Job drawing, mm, ordinate dimensions from the low corner. One solid piece. Give positions to 0.01 mm unless a question says otherwise; leave off trailing zeros. Order: outer loops, then holes, each group sorted by start corner. A loop starts at its lowest first (then second) coordinate and runs counter-clockwise, first axis right, second up. Notation, with made-up numbers: (-31.5, 50.25) - (16.5, 50.25) arc R7 cw to (16.5, 57.25) - close; hole circle Ø1 at (-38.5, 34). An arc over 180 degrees is marked (long way). Use one line per item in the form item = value. Start each with the question number.
1. Pull direction Z, two halves, no side cores. Call the marked faces 1, 2 and 3: +Z half, -Z half, draft (parallel to the pull), parting line (faces both ways), or undercut.
2. Pin check, flat tips, straight feed: P1, Ø2.5, axis at x = 3.5, z = 61, coming from the -Y side; P2, Ø3, axis at x = 163, y = 16, coming from the +Z side. Stop position of each tip, or through.
3. Band-saw the part on A-A, the plane z = 101. List the corners of the cut face in (x, y).
4. Band-saw the part on B-B, the plane x = 135.5. List the corners of the cut face in (y, z), plus the area to 3 significant figures.
5. Band-saw the part on D-D, the plane y = 12. List the corners of the cut face in (x, z) (1 decimal), plus the area to 3 significant figures.
6. Drill centre lines: line 1 (X direction, y = 41, z = 54.5); line 2 (Z direction, x = 31.5, y = 3); line 3 (X direction, y = 32, z = 14.5). Where is each one in solid material? Low to high.
7. Band-saw the part on C-C, the plane y = 42. List the corners of the cut face in (x, z).
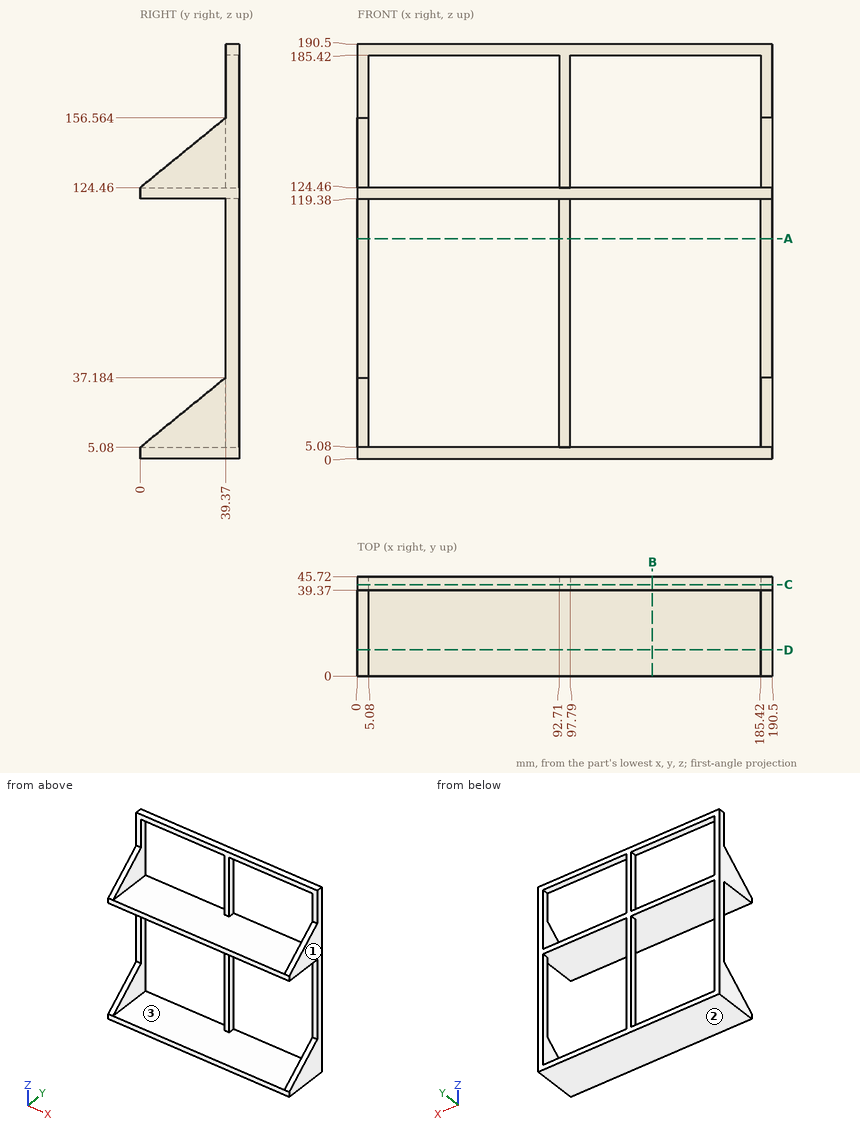
From the geometry:
q1.face_1 = draft
q1.face_2 = -Z half
q1.face_3 = undercut
q2.P1 = 39.37
q2.P2 = 124.46
q3.outline = (0, 39.37) - (5.08, 39.37) - (5.08, 45.72) - (0, 45.72) - close; (92.71, 39.37) - (97.79, 39.37) - (97.79, 45.72) - (92.71, 45.72) - close; (185.42, 39.37) - (190.5, 39.37) - (190.5, 45.72) - (185.42, 45.72) - close
q4.outline = (0, 0) - (45.72, 0) - (45.72, 5.08) - (0, 5.08) - close; (0, 119.38) - (45.72, 119.38) - (45.72, 124.46) - (0, 124.46) - close; (39.37, 185.42) - (45.72, 185.42) - (45.72, 190.5) - (39.37, 190.5) - close
q4.area = 497 mm²
q5.outline = (0, 0) - (190.5, 0) - (190.5, 14.9) - (185.4, 14.9) - (185.4, 5.1) - (5.1, 5.1) - (5.1, 14.9) - (0, 14.9) - close; (0, 119.4) - (190.5, 119.4) - (190.5, 134.2) - (185.4, 134.2) - (185.4, 124.5) - (5.1, 124.5) - (5.1, 134.2) - (0, 134.2) - close
q5.area = 2,130 mm²
q6.line_1 = 0 to 5.08, 92.71 to 97.79, 185.42 to 190.5
q6.line_2 = 0 to 5.08, 119.38 to 124.46
q6.line_3 = 0 to 5.08, 185.42 to 190.5
q7.outline = (0, 0) - (190.5, 0) - (190.5, 190.5) - (0, 190.5) - close; hole (5.08, 5.08) - (92.71, 5.08) - (92.71, 119.38) - (5.08, 119.38) - close; hole (5.08, 124.46) - (92.71, 124.46) - (92.71, 185.42) - (5.08, 185.42) - close; hole (97.79, 5.08) - (185.42, 5.08) - (185.42, 119.38) - (97.79, 119.38) - close; hole (97.79, 124.46) - (185.42, 124.46) - (185.42, 185.42) - (97.79, 185.42) - close
